Read the model definition and answer for the solid it produces. Units are mm, in the model's axes. Face numbers are marked on the shaded views. A direction names the side the tool comes from. Round coordinates to 2 decimals unless told otherwise and drop trailing zeros. Order: outer loops, then holes, each group sorted by start corner. A loop starts at its lowest first (then second) coordinate and runs counter-clockwise, first axis right, second up. Notation, with made-up numbers: (24, 44) - (40, 44) arc R24 cw to (40, 73) - close; hole circle Ø9 at (-2, 51.5). An arc over 180 degrees is marked (long way). Put each result on its own line as item: value. Start each with the question number.
Q1. Section C-C on x = 21 is taken. Give the vertices of the cut face in (y, z).
Q2. Section D-D on z = -15 is taken. Give the vertices of the cut face in (x, y), then the cut area to 3 significant figures.
Q3. Each of these flat-tipped pins is pushed along its axis until it touches: pin 1 Ø1.4 at (y, z) = (-4, 15) entering from -X; pin 2 Ø2.5 at (y, z) = (2, 1) entering from +X; pin 3 Ø1 at (y, z) = (1, -11.5) entering from -X; pin 4 Ø2.5 at (y, z) = (2, -4) entering from -X. Where does it stop, or does it pass through?
Q4. Find the intervals of material crossed by line 1 along Y through (x, z) = (-48, 15); line 2 along X through (y, z) = (-3, 16); line 3 along X through (y, z) = (2.5, 6), in increasing order. Write a range as from..to.
Q5. Section A-A on y = -7 is taken. Give the vertices of the cut face in (x, z), then the cut area to 3 significant figures.
Q6. For a pull along Z with two mould halves and no side action, classify the marked faces 3, 4, 5 and 6 as pulls with the +Z half, pulls with the -Z half, needs draft (parallel to the pull), parting line crosses it, or undercut.
Q7. Which of the six approach directions +Z, -Z, +X, -X, +Y, -Y give full straight-line access (tool end or side, diameter ignored) to the marked faces 1 and 2?
Q8. Section B-B on z = -6.5 is taken. Give the vertices of the cut face in (x, y), then the cut area to 3 significant figures.
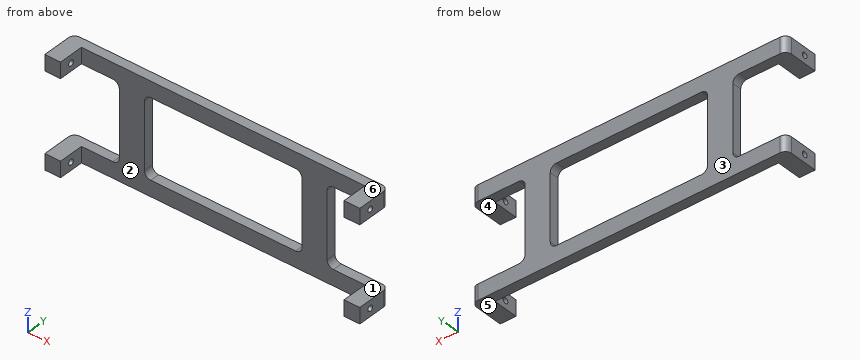
from build123d import *

# Parameters (mm, degrees)
SKETCH_1_W                  = 100
SKETCH_1_H                  = 35
EXTRUDE_1_DEPTH             = 3
SKETCH_2_W                  = 17
SKETCH_2_H                  = 25
CUT_EXTRUDE_1_DEPTH         = 54.058929503
SKETCH_3_W                  = 5
SKETCH_3_H                  = 5
EXTRUDE_2_DEPTH             = 8
SKETCH_4_W                  = 5
SKETCH_4_H                  = 5
EXTRUDE_3_DEPTH             = 8
SKETCH_5_W                  = 17
SKETCH_5_H                  = 30
CUT_EXTRUDE_2_DEPTH         = 54.574714185
SKETCH_6_W                  = 5
SKETCH_6_H                  = 5
EXTRUDE_4_DEPTH             = 8
SKETCH_7_W                  = 5
SKETCH_7_H                  = 3
EXTRUDE_5_DEPTH             = 17
SKETCH_8_W                  = 5
SKETCH_8_H                  = 5
EXTRUDE_6_DEPTH             = 8
SKETCH_9_W                  = 50
SKETCH_9_H                  = 25
CUT_EXTRUDE_3_DEPTH         = 55.104066391
HOLE_WIZARD_1_8_1_8_1_D     = 1.8
HOLE_WIZARD_1_8_1_8_1_DEPTH = 5
HOLE_WIZARD_1_8_1_8_2_D     = 1.8
HOLE_WIZARD_1_8_1_8_2_DEPTH = 100
FILLET_1_R                  = 2


with BuildPart() as part:
    # 草图1 → 凸台-拉伸1 (new body)
    with BuildSketch(Plane.XZ):
        Rectangle(SKETCH_1_W, SKETCH_1_H)
    extrude(amount=-EXTRUDE_1_DEPTH)

    # 草图2 → 切除-拉伸1 (cut, through all)
    with BuildSketch(Plane.XZ):
        with Locations((41.5, 0)):
            Rectangle(SKETCH_2_W, SKETCH_2_H)
    extrude(amount=-CUT_EXTRUDE_1_DEPTH, mode=Mode.SUBTRACT)

    # 草图3 → 凸台-拉伸2 (add)
    with BuildSketch(Plane.XZ):
        with Locations((47.5, -15)):
            Rectangle(SKETCH_3_W, SKETCH_3_H)
    extrude(amount=EXTRUDE_2_DEPTH)

    # 草图4 → 凸台-拉伸3 (add)
    with BuildSketch(Plane.XZ):
        with Locations((47.5, 15)):
            Rectangle(SKETCH_4_W, SKETCH_4_H)
    extrude(amount=EXTRUDE_3_DEPTH)

    # 草图5 → 切除-拉伸2 (cut, through all)
    with BuildSketch(Plane.XZ):
        with Locations((-41.5, 2.5)):
            Rectangle(SKETCH_5_W, SKETCH_5_H)
    extrude(amount=-CUT_EXTRUDE_2_DEPTH, mode=Mode.SUBTRACT)

    # 草图6 → 凸台-拉伸4 (add)
    with BuildSketch(Plane.XZ):
        with Locations((-47.5, -15)):
            Rectangle(SKETCH_6_W, SKETCH_6_H)
    extrude(amount=EXTRUDE_4_DEPTH)

    # 草图7 → 凸台-拉伸5 (add)
    with BuildSketch(Plane.ZY.offset(33)):
        with Locations((15, 1.5)):
            Rectangle(SKETCH_7_W, SKETCH_7_H)
    extrude(amount=EXTRUDE_5_DEPTH)

    # 草图8 → 凸台-拉伸6 (add)
    with BuildSketch(Plane.XZ):
        with Locations((-47.5, 15)):
            Rectangle(SKETCH_8_W, SKETCH_8_H)
    extrude(amount=EXTRUDE_6_DEPTH)

    # 草图9 → 切除-拉伸3 (cut, through all)
    with BuildSketch(Plane(origin=(0, 3, 0), x_dir=(-1, 0, 0), z_dir=(0, 1, 0))):
        Rectangle(SKETCH_9_W, SKETCH_9_H)
    extrude(amount=-CUT_EXTRUDE_3_DEPTH, mode=Mode.SUBTRACT)

    # Ø1.8 (1.8) 直径孔1
    with Locations(Plane.ZY.offset(50)):
        with Locations((15, -4), (-15, -4)):
            Hole(HOLE_WIZARD_1_8_1_8_1_D / 2, depth=HOLE_WIZARD_1_8_1_8_1_DEPTH)

    # Ø1.8 (1.8) 直径孔2
    with Locations(Plane(origin=(50, 0, 0), x_dir=(0, 0, -1), z_dir=(1, 0, 0))):
        with Locations((15, -4), (-15, -4)):
            Hole(HOLE_WIZARD_1_8_1_8_2_D / 2, depth=HOLE_WIZARD_1_8_1_8_2_DEPTH)

    # 圆角1
    fillet_1_edges = [part.edges().sort_by_distance(p)[0] for p in [
        (-25, 1.5, -12.5),
        (25, 1.5, -12.5),
        (25, 1.5, 12.5),
        (-25, 1.5, 12.5),
        (50, 3, 15),
        (33, 1.5, -12.5),
        (33, 1.5, 12.5),
        (50, 3, -15),
        (-50, 3, -15),
        (-33, 1.5, -12.5),
        (-33, 1.5, 12.5),
        (-50, 3, 15),
    ]]
    fillet(fillet_1_edges, radius=FILLET_1_R)


solid = part.part
Findings:
1. outline: (0, -17.5) - (3, -17.5) - (3, -12.5) - (0, -12.5) - close; (0, 12.5) - (3, 12.5) - (3, 17.5) - (0, 17.5) - close
2. outline: (-50, -8) - (-45, -8) - (-45, -4.9) - (-50, -4.9) - close; (-50, -3.1) - (-45, -3.1) - (-45, 0) - (45, 0) - (45, -3.1) - (50, -3.1) - (50, 1) arc R2 ccw to (48, 3) - (-48, 3) arc R2 ccw to (-50, 1) - close; (45, -8) - (50, -8) - (50, -4.9) - (45, -4.9) - close
2. area: 360 mm2
3. pin 1: through
3. pin 2: x = 33
3. pin 3: x = -33.68
3. pin 4: x = -33
4. line 1: -8..-4.9, -3.1..3
4. line 2: -50..-45, 45..50
4. line 3: -33..-25, 25..33
5. outline: (-50, -17.5) - (-45, -17.5) - (-45, -12.5) - (-50, -12.5) - close; (-50, 12.5) - (-45, 12.5) - (-45, 17.5) - (-50, 17.5) - close; (45, -17.5) - (50, -17.5) - (50, -12.5) - (45, -12.5) - close; (45, 12.5) - (50, 12.5) - (50, 17.5) - (45, 17.5) - close
5. area: 100 mm2
6. face 3: needs draft
6. face 4: undercut
6. face 5: pulls with the -Z half
6. face 6: pulls with the +Z half
7. face 1: +X, +Y, -Y
7. face 2: +Z, -Z, -Y
8. outline: (-33, 0) - (-25, 0) - (-25, 3) - (-33, 3) - close; (25, 0) - (33, 0) - (33, 3) - (25, 3) - close
8. area: 48.0 mm2
